Design review of the part built by this model. Coordinates are the model's own, in mm. A direction names the side the tool comes from. Give positions to 0.01 mm unless a question says otherwise; leave off trailing zeros. Order: outer loops, then holes, each group sorted by start corner. A loop starts at its lowest first (then second) coordinate and runs counter-clockwise, first axis right, second up. Notation, with made-up numbers: M 85,87.5 L 121,87.5 A24 ccw 121,114.5 Z; hole C 66.25,33.25 d10. An arc over 180 degrees is marked long. Answer as a JSON object with one key per item and string values.
from build123d import *

# Parameters (mm, degrees)
EXTRUDE_THIN1_DEPTH = 362.7
FILLET1_R           = 3


with BuildPart() as part:
    # Sketch1 → Extrude-Thin1 (new body)
    with BuildSketch(Plane.XY):
        Polygon((0, 0), (0, -100), (165, -145), (535, -145), (700, -55), (700, 0), (701.5875, 0), (701.5875, -55.942392544), (535.404802998, -146.5875), (164.787405042, -146.5875), (-1.5875, -101.212525898), (-1.5875, 0), align=None)
    extrude(amount=EXTRUDE_THIN1_DEPTH)

    # Fillet1
    fillet1_edges = [part.edges().sort_by_distance(p)[0] for p in [
        (700, -55, 181.35),
        (535, -145, 181.35),
        (165, -145, 181.35),
        (0, -100, 181.35),
        (-1.5875, -101.212525898, 181.35),
        (164.787405042, -146.5875, 181.35),
        (535.404802998, -146.5875, 181.35),
        (701.5875, -55.942392544, 181.35),
    ]]
    fillet(fillet1_edges, radius=FILLET1_R)


solid = part.part
(1) We need section B-B (y = -69). Write out the cut boundary in (x, z), plus the area to 3 significant figures.
Checked values:
{"outline": "M -1.59,0 L 0,0 L 0,362.7 L -1.59,362.7 Z; M 674.33,0 L 677.65,0 L 677.65,362.7 L 674.33,362.7 Z", "area": "1,780 mm^2"}
(2) We need section A-A (z = 230.5). Write out the cut boundary in (x, y).
Checked values:
{"outline": "M -1.59,-98.92 A3 ccw 0.62,-101.82 L 164.4,-146.48 A3 ccw 165.19,-146.59 L 534.64,-146.59 A3 ccw 536.08,-146.22 L 700.02,-56.8 A3 ccw 701.59,-54.16 L 701.59,0 L 700,0 L 700,-53.22 A3 cw 698.44,-55.85 L 535.67,-144.63 A3 cw 534.24,-145 L 165.4,-145 A3 cw 164.61,-144.89 L 2.21,-100.6 A3 cw 0,-97.71 L 0,0 L -1.59,0 Z"}
(3) We need section C-C (x = 362.5). Write out the cut boundary in (y, z).
Checked values:
{"outline": "M -146.59,0 L -145,0 L -145,362.7 L -146.59,362.7 Z"}
(4) To check wall thickness, follow L1, parallel to X at y = -52.5, z = 340.5; L2, parallel to Y at x = 313, z = 109.5; L3, parallel to X at y = -71, z = 149. State the ranges of each line that lie inside material, in increasing order. Write a range as from..to.
Checked values:
{"L1": "x = -1.59..0, 700..701.59", "L2": "y = -146.59..-145", "L3": "x = -1.59..0, 670.67..673.98"}
(5) We need section D-D (y = -117.5). Write out the cut boundary in (x, z), plus the area to 3 significant figures.
Checked values:
{"outline": "M 58.13,0 L 64.17,0 L 64.17,362.7 L 58.13,362.7 Z; M 585.42,0 L 588.73,0 L 588.73,362.7 L 585.42,362.7 Z", "area": "3,390 mm^2"}
(6) Insertion check: pin 1 (1.5 mm diameter, centred on y = -95.5, z = 62.5, fed in from +X); pin 2 (1 mm diameter, centred on y = -130.5, z = 240, fed in from +X); pin 3 (8 mm diameter, centred on y = -98.5, z = 171.5, fed in from +X); pin 4 (10 mm diameter, centred on x = 95.5, y = -116.5, fed in from -Z). Each pin has a flat end and moves straight along its axis. Give the tip position at first contact, or say it passes through.
Checked values:
{"pin 1": "stops at x = 630.44", "pin 2": "stops at x = 565.82", "pin 3": "stops at x = 630.9", "pin 4": "passes through"}
(7) Tool access review of faces 4 (the flat face through (615.915, -100.865, 178.811)), 5 (the flat face through (353, -146.588, 179)): name each direction out of +Z, -Z, +X, -X, +Y, -Y from which nothing blocks a thin tool from reaching the whole face with its end or side.
Checked values:
{"face 4": "+Z, -Z, +Y", "face 5": "+Z, -Z, +X, -X, -Y"}
(8) Draft analysis for pull direction X (two halves, no side actions). For faces 1 (the flat face through (0, -48, 179)), 2 (the flat face through (-1.588, -50, 179)), 3 (the flat face through (701.588, -27, 179)), state which applies: +X half, -X half, draft (parallel to the pull), parting line (faces both ways), or undercut.
Checked values:
{"face 1": "undercut", "face 2": "-X half", "face 3": "+X half"}
